from build123d import *

# Parameters (mm, degrees)
F0_W      = 72.39
F0_H      = 138.684
F1_DEPTH  = 1.905
F2_W      = 72.39
F2_H      = 138.684
F2_W_2    = 67.31
F2_H_2    = 133.604
F3_DEPTH  = 10.668
F4_W      = 25.4
F4_H      = 25.4
F5_DEPTH  = 1.905
F6_W      = 6.35
F6_H      = 12.573
F7_DEPTH  = 3.175
F8_W      = 3.175
F8_H      = 12.573
F9_DEPTH  = 38.1
F10_W     = 3.175
F10_H     = 25.4
F11_DEPTH = 12.573
F12_W     = 72.39
F12_H     = 25.4
F13_DEPTH = 12.574


with BuildPart() as f1:
    # F0 (on Top) → F1 (new body)
    with BuildSketch(Plane.XY):
        with Locations((36.195, 69.342)):
            Rectangle(F0_W, F0_H)
    extrude(amount=F1_DEPTH)

    # F2 (on face) → F3 (join)
    with BuildSketch(Plane.XY.offset(1.905)):
        with Locations((36.195, 69.342)):
            Rectangle(F2_W, F2_H)
        with Locations((36.195, 69.342)):
            Rectangle(F2_W_2, F2_H_2, mode=Mode.SUBTRACT)
    extrude(amount=F3_DEPTH)

    # F4 (on face) → F5 (cut, through all)
    with BuildSketch(Plane(origin=(0, 0, 0), x_dir=(1, 0, 0), z_dir=(0, 0, -1))):
        with Locations((36.195, -120.904)):
            Rectangle(F4_W, F4_H)
    extrude(amount=-F5_DEPTH, mode=Mode.SUBTRACT)

    # F6 (on face) → F7 (join)
    with BuildSketch(Plane.YZ.offset(72.39)):
        with Locations((53.467, 6.2865)):
            Rectangle(F6_W, F6_H)
        with Locations((85.217, 6.2865)):
            Rectangle(F6_W, F6_H)
    extrude(amount=F7_DEPTH)

    # F8 (on face) → F9 (join, through all)
    with BuildSketch(Plane.XZ.offset(-50.292)):
        with Locations((77.1525, 6.2865)):
            Rectangle(F8_W, F8_H)
    extrude(amount=-F9_DEPTH)

    # F10 (on face) → F11 (join, through all)
    with BuildSketch(Plane.XY.offset(12.573)):
        Polygon((0, 82.042), (0, 88.392), (-6.35, 88.392), (-6.35, 82.042), (-3.175, 82.042), align=None)
        with Locations((-4.7625, 69.342)):
            Rectangle(F10_W, F10_H)
        Polygon((-3.175, 56.642), (-6.35, 56.642), (-6.35, 50.292), (0, 50.292), (0, 56.642), align=None)
    extrude(amount=-F11_DEPTH)

    # F12 (on face) → F13 (cut, through all)
    with BuildSketch(Plane(origin=(0, 0, 0), x_dir=(1, 0, 0), z_dir=(0, 0, -1))):
        with Locations((36.195, -12.7)):
            Rectangle(F12_W, F12_H)
    extrude(amount=-F13_DEPTH, mode=Mode.SUBTRACT)


solid = f1.part
Input: part model. Units: mm. Frame: model coordinates. A direction names the side the tool comes from. Give positions to 0.01 mm unless a question says otherwise; leave off trailing zeros. Write each loop counter-clockwise with the first axis right and the second up, starting at its lowest first coordinate (ties: lowest second). Pieces come first, ordered by that corner, then holes.
Q1. Section A-A, the plane y = 59.5. Output: boundary loops of the cut face in (x, z) (3 decimals).
Q2. Section B-B, the plane x = 32. Output: boundary loops of the cut face in (y, z) (3 decimals), plus the area to 3 significant figures.
Q3. Pull-direction query (X, two-part tool) for faces 5 (the face through (36, 81, 0)), 6 (the face through (-3.175, 69, 6)), 7 (the face through (0, 113, 6)), 8 (the face through (36, 82, 1.905)); classes: pulls with the +X half, pulls with the -X half, needs draft (parallel to the pull), parting line crosses it, or undercut.
Q4. Section D-D, the plane y = 124. Output: boundary loops of the cut face in (x, z) (3 decimals), plus the area to 3 significant figures.
Q5. First-contact query: P1, Ø5, axis at x = -1.5, z = 5, coming from the +Y side; P2, Ø1.5, axis at y = 122.5, z = 1.5, coming from the +X side; P3, Ø1, axis at x = 7, y = 38.5, coming from the +Z side (3 decimals); P4, Ø1.9, axis at x = 75, z = 5.5, coming from the -Y side. Flat tips, straight axial feed; report the tip coordinate or a pass-through.
Q6. Section C-C, the plane z = 9. Output: boundary loops of the cut face in (x, y) (3 decimals).
Q7. Set-up query: faces 1 (the face through (36, 136.144, 7)), 2 (the face through (74, 56.642, 6)), 3 (the face through (-3, 88.392, 6)), 4 (the face through (76, 50.292, 6)). Return all of +Z, -Z, +X, -X, +Y, -Y with unobstructed straight access to the full face (end or side cutting, diameter ignored); none if empty.
Q8. Material intervals for probe 1 along X at (y, z) = (57, 8.25) (3 decimals); probe 2 along X at (y, z) = (80, 1) (3 decimals); probe 3 along X at (y, z) = (90.5, 7.5), sorted ascending.
Filled in:
1. outline: (-6.35, 0) - (-3.175, 0) - (-3.175, 12.573) - (-6.35, 12.573) - close; (0, 0) - (72.39, 0) - (72.39, 12.573) - (69.85, 12.573) - (69.85, 1.905) - (2.54, 1.905) - (2.54, 12.573) - (0, 12.573) - close; (75.565, 0) - (78.74, 0) - (78.74, 12.573) - (75.565, 12.573) - close
2. outline: (25.4, 0) - (108.204, 0) - (108.204, 1.905) - (25.4, 1.905) - close; (133.604, 0) - (138.684, 0) - (138.684, 12.573) - (136.144, 12.573) - (136.144, 1.905) - (133.604, 1.905) - close
2. area: 195 mm2
3. face 5: needs draft
3. face 6: undercut
3. face 7: pulls with the -X half
3. face 8: undercut
4. outline: (0, 0) - (23.495, 0) - (23.495, 1.905) - (2.54, 1.905) - (2.54, 12.573) - (0, 12.573) - close; (48.895, 0) - (72.39, 0) - (72.39, 12.573) - (69.85, 12.573) - (69.85, 1.905) - (48.895, 1.905) - close
4. area: 144 mm2
5. P1: stops at y = 138.68
5. P2: stops at x = 72.39
5. P3: stops at z = 1.905
5. P4: stops at y = 50.29
6. outline: (-6.35, 50.292) - (0, 50.292) - (0, 25.4) - (2.54, 25.4) - (2.54, 136.144) - (69.85, 136.144) - (69.85, 25.4) - (72.39, 25.4) - (72.39, 50.292) - (78.74, 50.292) - (78.74, 88.392) - (72.39, 88.392) - (72.39, 138.684) - (0, 138.684) - (0, 88.392) - (-6.35, 88.392) - close; hole (-3.175, 56.642) - (0, 56.642) - (0, 82.042) - (-3.175, 82.042) - close; hole (72.39, 56.642) - (75.565, 56.642) - (75.565, 82.042) - (72.39, 82.042) - close
7. face 1: +Z, -Y
7. face 2: +Z, -Z
7. face 3: +Z, -Z, -X, +Y
7. face 4: +Z, -Z, +X, -Y
8. probe 1: x = -6.35 to -3.175, 0 to 2.54, 69.85 to 72.39, 75.565 to 78.74
8. probe 2: x = -6.35 to -3.175, 0 to 72.39, 75.565 to 78.74
8. probe 3: x = 0 to 2.54, 69.85 to 72.39
